Design review of the part built by this model. Coordinates are the model's own, in mm. A direction names the side the tool comes from. Coordinates: 2 decimals unless noted, no trailing zeros. Write each loop counter-clockwise with the first axis right and the second up, starting at its lowest first coordinate (ties: lowest second). Pieces come first, ordered by that corner, then holes. Notation, with made-up numbers: (-21, -8) - (1, -8) arc R10 ccw to (1, 10) - close; hole circle Ø5 at (-10.5, 29.5). An arc over 180 degrees is marked (long way). Answer as CSV lines item,"result". Start each with the question number.
Q1. For line 1 along Y through (x, z) = (0, 33) (3 decimals); line 2 along Z through (x, y) = (49.5, 15.5); line 3 along Y through (x, z) = (-6, 35), list the stretches that pass through material, from the lowest coordinate up. Write a range as [from, to].
Q2. Machinability: for faces 5 (the face through (63, 13, 14.288)), 6 (the face through (86.04, 12.79, 41.73)), 7 (the face through (57, 6.35, 12)), which of the approach directions +Z, -Z, +X, -X, +Y, -Y give a long, thin tool a straight path to every point of the face, cutting with its end or side? Answer none if there is none.
Q3. Mouldability with a two-part tool opening along Y and no side actions: class faces 1 (the face through (19, 5, 44.45)), 2 (the face through (45, 19.05, 12)), 3 (the face through (-7.559, -5.796, 21.914)), 4 (the face through (-13.907, -13.019, 21.914)) as pulls with the +Y half, pulls with the -Y half, needs draft (parallel to the pull), parting line crosses it, or undercut.
Q4. We need section C-C (z = 40.5). Write out the cut boundary in (x, y) (3 decimals).
Q5. We need section B-B (y = -3.5). Write out the cut boundary in (x, z).
Q6. We need section A-A (x = 36.5). Write out the cut boundary in (y, z), plus the area to 3 significant figures.
Q7. Clearance check with flat-ended pins moving along their axes: pin 1 (1.5 mm diameter, centred on y = 4, z = 34, fed in from -X); pin 2 (22 mm diameter, centred on x = 45.5, z = 18, fed in from -Y); pin 3 (1 mm diameter, centred on y = 1.5, z = 34, fed in from +X). State where each tip first meets the part, or that it passes through.
Q8. We need section D-D (x = 15.5). Write out the cut boundary in (y, z).
from build123d import *

# Parameters (mm, degrees)
F0_R        = 9.525
F1_DEPTH    = 44.45
F2_W        = 50.8
F2_H        = 15.875
F4_DEPTH    = 12.7
F5_R        = 9.525
F6_T1_DEPTH = 44.45


# Not quite as in the source:
# - a fillet or chamfer that OpenCascade refuses, or shapes differently, is made with other operations: its cross-section is extruded or revolved along the edge and cut away or added
# - a length typed as a fraction of an inch, garbled in the dataset ("3 / 203.2 mm" for 3/8 in), is restored


with BuildPart() as f1:
    # F0 (on Top) → F1 (new body)
    with BuildSketch(Plane.XY):
        with BuildLine():
            ThreePointArc((0, 19.05), (-13.4703841816, -13.4703841816), (19.05, 0))
            ThreePointArc((19.05, 0), (18.7756525614, 3.2213926947), (17.9605122421, 6.35))
            ThreePointArc((17.9605122421, 6.35), (10.9985226281, 15.5542598667), (0, 19.05))
        make_face()
        Circle(F0_R, mode=Mode.SUBTRACT)
        with BuildLine():
            ThreePointArc((0, 19.05), (10.9985226281, 15.5542598667), (17.9605122421, 6.35))
            Line((17.9605122421, 6.35), (88.9, 6.35))
            Line((88.9, 6.35), (88.9, 19.05))
            Line((88.9, 19.05), (0, 19.05))
        make_face()
    extrude(amount=F1_DEPTH)

    # F3 (on face) + F2 (on face) → F4 (cut)
    with BuildSketch(Plane.XZ.offset(-6.35)):
        with BuildLine():
            Line((38.1, 14.2883619165), (38.1, 30.1616380835))
            ThreePointArc((38.1, 30.1616380835), (30.279470861, 22.225), (38.1, 14.2883619165))
        make_face()
    with BuildSketch(Plane.XZ.offset(-6.35)):
        with Locations((63.5, 22.225)):
            Rectangle(F2_W, F2_H)
    extrude(amount=-F4_DEPTH, mode=Mode.SUBTRACT)

    # F5
    f5_edges = [f1.edges().sort_by_distance(p)[0] for p in [
        (88.9, 12.7, 44.45),
        (88.9, 12.7, 0),
    ]]
    fillet(f5_edges, radius=F5_R)

    # F6: fillet of radius 6.35 on 1 edges, made by hand

    # F6_s2 → F6_t1 (join)
    with BuildSketch(Plane.XY):
        with BuildLine():
            ThreePointArc((19.05, 0), (20.9098719395, 4.4901280605), (25.4, 6.35))
            Line((25.4, 6.35), (17.9605122421, 6.35))
            ThreePointArc((17.9605122421, 6.35), (18.7756525614, 3.2213926947), (19.05, 0))
        make_face()
    extrude(amount=F6_T1_DEPTH)


solid = f1.part
Results list:
1,line 1,"y = [-19.05, -9.525], [9.525, 19.05]"
1,line 2,"z = [0, 14.29], [30.16, 44.45]"
1,line 3,"y = [-18.08, -7.4], [7.4, 18.08]"
2,face 5,"+X, +Y, -Y"
2,face 6,"+Z, +X, +Y, -Y"
2,face 7,"+Z, -Z, +X, -Y"
3,face 1,"needs draft"
3,face 2,"pulls with the +Y half"
3,face 3,"undercut"
3,face 4,"parting line crosses it"
4,outline,"(0, 19.05) arc R19.05 ccw (long way) to (19.05, 0) arc R6.35 cw to (25.4, 6.35) - (87.098, 6.35) - (87.098, 19.05) - close; hole circle Ø19.05 at (0, 0)"
5,outline,"(-18.73, 0) - (-8.86, 0) - (-8.86, 44.45) - (-18.73, 44.45) - close; (8.86, 0) - (18.73, 0) - (18.73, 44.45) - (8.86, 44.45) - close"
6,outline,"(6.35, 0) - (19.05, 0) - (19.05, 14.48) - (6.35, 14.48) - close; (6.35, 29.97) - (19.05, 29.97) - (19.05, 44.45) - (6.35, 44.45) - close"
6,area,"368 mm2"
7,pin 1,"stops at x = -18.77"
7,pin 2,"stops at y = 6.35"
7,pin 3,"stops at x = 19.37"
8,outline,"(-11.07, 0) - (19.05, 0) - (19.05, 44.45) - (-11.07, 44.45) - close"
